```python
from build123d import *

# Parameters (mm, degrees)
SKETCH1_W           = 317.5
SKETCH1_H           = 152.4
BOSS_EXTRUDE1_DEPTH = 76.2
SKETCH2_W           = 302.26
SKETCH2_H           = 137.16
CUT_EXTRUDE1_DEPTH  = 68.58
CUT_EXTRUDE2_REACH  = 319.5
BOSS_EXTRUDE2_DEPTH = 25.4
CUT_EXTRUDE3_REACH  = 9.62
SKETCH7_R           = 3
BOSS_EXTRUDE4_DEPTH = 7.62
FILLET2_R           = 12.7
FILLET3_R           = 2.54


with BuildPart() as part:
    # Sketch1 → Boss-Extrude1 (new body)
    with BuildSketch(Plane.XY):
        Rectangle(SKETCH1_W, SKETCH1_H)
    extrude(amount=BOSS_EXTRUDE1_DEPTH)

    # Sketch2 → Cut-Extrude1 (cut)
    with BuildSketch(Plane(origin=(0, 0, 0), x_dir=(-1, 0, 0), z_dir=(0, 0, -1))):
        Rectangle(SKETCH2_W, SKETCH2_H)
    extrude(amount=-CUT_EXTRUDE1_DEPTH, mode=Mode.SUBTRACT)

    # Sketch3 → Cut-Extrude2 (cut, up to next)
    with BuildSketch(Plane.ZY.offset(158.75), mode=Mode.PRIVATE) as cut_extrude2_sk1:
        with BuildLine():
            Line((42.037, 38.5445), (0, 38.5445))
            Line((0, 38.5445), (0, 45.5295))
            Line((0, 45.5295), (42.037, 45.5295))
            ThreePointArc((42.037, 45.5295), (45.5295, 42.037), (42.037, 38.5445))
        make_face()
    cut_extrude2_tool1 = extrude(cut_extrude2_sk1.sketch, amount=-CUT_EXTRUDE2_REACH, mode=Mode.PRIVATE) & part.part
    add(cut_extrude2_tool1.solids().sort_by_distance((-158.75, 42.037, 22.396786))[0], mode=Mode.SUBTRACT)

    # Sketch4 → Boss-Extrude2 (add)
    with BuildSketch(Plane(origin=(0, 0, 68.58), x_dir=(-1, 0, 0), z_dir=(0, 0, -1))):
        Polygon((-151.13, 0), (0, 0), (0, -68.58), (-7.112, -68.58), (-7.112, -6.35), (-151.13, -6.35), align=None)
    extrude(amount=BOSS_EXTRUDE2_DEPTH)

    # Sketch5 → Cut-Extrude3 (cut, up to next)
    with BuildSketch(Plane.ZY.offset(-151.13), mode=Mode.PRIVATE) as cut_extrude3_sk1:
        with BuildLine():
            Line((5.08, 38.5445), (0, 38.5445))
            Line((0, 38.5445), (0, 45.5295))
            Line((0, 45.5295), (5.08, 45.5295))
            ThreePointArc((5.08, 45.5295), (8.5725, 42.037), (5.08, 38.5445))
        make_face()
    cut_extrude3_tool1 = extrude(cut_extrude3_sk1.sketch, amount=-CUT_EXTRUDE3_REACH, mode=Mode.PRIVATE) & part.part
    add(cut_extrude3_tool1.solids().sort_by_distance((151.13, 42.037, 3.950338))[0], mode=Mode.SUBTRACT)

    # Sketch7 → Boss-Extrude4 (add)
    with BuildSketch(Plane(origin=(0, 0, 68.58), x_dir=(-1, 0, 0), z_dir=(0, 0, -1))):
        with Locations((140.01, -63.81)):
            Circle(SKETCH7_R)
        with Locations((82.01, -63.81)):
            Circle(SKETCH7_R)
        with Locations((140.01, -14.81)):
            Circle(SKETCH7_R)
        with Locations((82.01, -14.81)):
            Circle(SKETCH7_R)
    extrude(amount=BOSS_EXTRUDE4_DEPTH)

    # Fillet2
    fillet2_edges = [part.edges().sort_by_distance(p)[0] for p in [
        (-151.13, 68.58, 34.29),
        (151.13, 68.58, 34.29),
        (151.13, -68.58, 34.29),
        (-151.13, -68.58, 34.29),
        (-158.75, 76.2, 38.1),
        (158.75, 76.2, 38.1),
        (158.75, -76.2, 38.1),
        (-158.75, -76.2, 38.1),
    ]]
    fillet(fillet2_edges, radius=FILLET2_R)

    # Fillet3
    fillet3_edges = [part.edges().sort_by_distance(p)[0] for p in [
        (151.13, 0, 55.88),
        (151.13, -6.35, 55.88),
        (7.112, -6.35, 55.88),
        (7.112, -68.58, 55.88),
        (0, -68.58, 55.88),
        (0, 0, 55.88),
        (151.13, -3.175, 43.18),
        (3.556, -68.58, 43.18),
    ]]
    fillet(fillet3_edges, radius=FILLET3_R)


solid = part.part
```
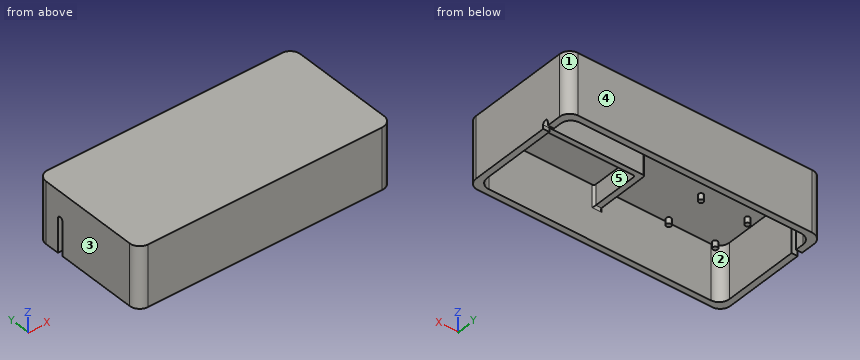
For this review, take the finished solid that the model builds, in its own axes (mm). Face numbers are marked on the shaded views. A direction names the side the tool comes from. Coordinates: 2 decimals unless noted, no trailing zeros. Loops run counter-clockwise (first coordinate to the right, second up) from the corner with the lowest first, then second, coordinate; pieces in that order, holes last.
1. Add section D-D, the plane y = -14.81. Give the boundary of the cut face in (x, z), then the cut area to 3 significant figures.
2. Mouldability with a two-part tool opening along Y and no side actions: class the marked faces 3, 4 and 5 as +Y half, -Y half, draft (parallel to the pull), parting line (faces both ways), or undercut.
3. For line 1 (Y direction, x = 102, z = 51); line 2 (X direction, y = -55, z = 68); line 3 (X direction, y = 51, z = 56.5), list the stretches that pass through material, from the lowest coordinate up.
4. Add section C-C, the plane x = -82.01. Give the boundary of the cut face in (y, z).
5. Add section B-B, the plane z = 51. Give the boundary of the cut face in (x, y).
6. Add section A-A, the plane z = 64. Count the separate pieces of the cut face and the enclosed holes in it, then the cut area to 3 significant figures.
7. Insertion check: P1, Ø10, axis at x = -9.5, y = -7, coming from the -Z side; P2, Ø6.5, axis at x = -82.5, y = -63.5, coming from the -Z side; P3, Ø5.5, axis at x = 154.5, z = 2.5, coming from the +Y side. Each pin has a flat end and moves straight along its axis. Give the tip position at first contact, or say it passes through.
8. For the marked faces 1 and 2, list the 3-axis set-ups (+Z, -Z, +X, -X, +Y, -Y) from which the entire face can be reached by the end or side of a thin tool; tool diameter is ignored.
Result:
1. outline: (-158.75, 0) - (-151.13, 0) - (-151.13, 68.58) - (-143.01, 68.58) - (-143.01, 60.96) - (-137.01, 60.96) - (-137.01, 68.58) - (-85.01, 68.58) - (-85.01, 60.96) - (-79.01, 60.96) - (-79.01, 68.58) - (0, 68.58) - (0, 43.18) - (7.11, 43.18) - (7.11, 68.58) - (151.13, 68.58) - (151.13, 0) - (158.75, 0) - (158.75, 76.2) - (-158.75, 76.2) - close
1. area: 3,740 mm2
2. face 3: draft
2. face 4: +Y half
2. face 5: undercut
3. line 1: y = -76.2 to -68.58, -6.35 to 0, 68.58 to 76.2
3. line 2: x = -158.75 to -151.13, 0 to 7.11, 151.13 to 158.75
3. line 3: x = -158.75 to -151.13, 151.13 to 158.75
4. outline: (-76.2, 0) - (-68.58, 0) - (-68.58, 68.58) - (-66.81, 68.58) - (-66.81, 60.96) - (-60.81, 60.96) - (-60.81, 68.58) - (-17.81, 68.58) - (-17.81, 60.96) - (-11.81, 60.96) - (-11.81, 68.58) - (68.58, 68.58) - (68.58, 0) - (76.2, 0) - (76.2, 76.2) - (-76.2, 76.2) - close
5. outline: (-158.75, -63.5) arc R12.7 ccw to (-146.05, -76.2) - (146.05, -76.2) arc R12.7 ccw to (158.75, -63.5) - (158.75, 63.5) arc R12.7 ccw to (146.05, 76.2) - (-146.05, 76.2) arc R12.7 ccw to (-158.75, 63.5) - close; hole (-151.13, -55.88) arc R12.7 ccw to (-138.43, -68.58) - (-2.54, -68.58) arc R2.54 ccw to (0, -66.04) - (0, -2.54) arc R2.54 cw to (2.54, 0) - (148.59, 0) arc R2.54 ccw to (151.13, 2.54) - (151.13, 55.88) arc R12.7 ccw to (138.43, 68.58) - (-138.43, 68.58) arc R12.7 ccw to (-151.13, 55.88) - close; hole (7.11, -66.04) arc R2.54 ccw to (9.65, -68.58) - (138.43, -68.58) arc R12.7 ccw to (151.13, -55.88) - (151.13, -8.89) arc R2.54 ccw to (148.59, -6.35) - (9.65, -6.35) arc R2.54 ccw to (7.11, -8.89) - close
6. separate pieces: 5
6. enclosed holes: 2
6. area: 8,450 mm2
7. P1: stops at z = 68.58
7. P2: stops at z = 60.96
7. P3: stops at y = 74.85
8. face 1: +Z, -Z, +X, +Y
8. face 2: -Z
